```python
from build123d import *

# Parameters (mm, degrees)
SKETCH1_W           = 228.6
SKETCH1_H           = 149.86
SKETCH1_R           = 2.54
SKETCH1_R_2         = 2.159
SKETCH1_W_2         = 25.4
SKETCH1_H_2         = 3.175
BOSS_EXTRUDE1_DEPTH = 2.6
FILLET1_R           = 10
SKETCH6_R           = 2.159
CUT_EXTRUDE6_DEPTH  = 2.6
SKETCH15_R          = 10
CUT_EXTRUDE14_DEPTH = 274.354604132
SKETCH25_W          = 104.14
SKETCH25_H          = 22.86
SKETCH25_W_2        = 3.2385
SKETCH25_H_2        = 12.7
CUT_EXTRUDE18_DEPTH = 10.16


with BuildPart() as part:
    # Sketch1 → Boss-Extrude1 (new body)
    with BuildSketch(Plane(origin=(0, 0, 0), x_dir=(1, 0, 0), z_dir=(0, 1, 0))):
        with Locations((114.3, -74.93)):
            Rectangle(SKETCH1_W, SKETCH1_H)
        with Locations(Location((5.08, -57.785, 0), (0, 0, 270))):
            Circle(SKETCH1_R, mode=Mode.SUBTRACT)
        with Locations(Location((5.08, -92.075, 0), (0, 0, 270))):
            Circle(SKETCH1_R, mode=Mode.SUBTRACT)
        with Locations(Location((223.52, -92.075, 0), (0, 0, 270))):
            Circle(SKETCH1_R, mode=Mode.SUBTRACT)
        with Locations(Location((223.52, -57.785, 0), (0, 0, 270))):
            Circle(SKETCH1_R, mode=Mode.SUBTRACT)
        with Locations(Location((218.44, -10.16, 0), (0, 0, 270))):
            Circle(SKETCH1_R_2, mode=Mode.SUBTRACT)
        with Locations(Location((10.16, -10.16, 0), (0, 0, 270))):
            Circle(SKETCH1_R_2, mode=Mode.SUBTRACT)
        with Locations(Location((218.44, -139.7, 0), (0, 0, 270))):
            Circle(SKETCH1_R_2, mode=Mode.SUBTRACT)
        with Locations(Location((10.16, -139.7, 0), (0, 0, 270))):
            Circle(SKETCH1_R_2, mode=Mode.SUBTRACT)
        with Locations((35.56, -9.887961988)):
            Rectangle(SKETCH1_W_2, SKETCH1_H_2, mode=Mode.SUBTRACT)
        with Locations((193.04, -9.887961988)):
            Rectangle(SKETCH1_W_2, SKETCH1_H_2, mode=Mode.SUBTRACT)
        with Locations((193.04, -139.972038012)):
            Rectangle(SKETCH1_W_2, SKETCH1_H_2, mode=Mode.SUBTRACT)
        with Locations((35.56, -139.972038012)):
            Rectangle(SKETCH1_W_2, SKETCH1_H_2, mode=Mode.SUBTRACT)
    extrude(amount=BOSS_EXTRUDE1_DEPTH)

    # Fillet1
    fillet1_edges = [part.edges().sort_by_distance(p)[0] for p in [
        (0, 1.3, 0),
        (228.6, 1.3, 0),
        (228.6, 1.3, 149.86),
        (0, 1.3, 149.86),
    ]]
    fillet(fillet1_edges, radius=FILLET1_R)

    # Sketch6 → Cut-Extrude6 (cut)
    with BuildSketch(Plane.XZ):
        with Locations((218.6, 10)):
            Circle(SKETCH6_R)
    extrude(amount=-CUT_EXTRUDE6_DEPTH, mode=Mode.SUBTRACT)

    # Sketch15 → Cut-Extrude14 (cut, through all)
    with BuildSketch(Plane.XZ):
        with Locations(Location((114.3, 74.93, 0), (0, 0, 270))):
            Circle(SKETCH15_R)
    extrude(amount=-CUT_EXTRUDE14_DEPTH, mode=Mode.SUBTRACT)

    # Sketch25 → Cut-Extrude18 (cut)
    with BuildSketch(Plane(origin=(0, 2.6, 0), x_dir=(1, 0, 0), z_dir=(0, 1, 0))):
        with Locations((114.3, -74.93)):
            Rectangle(SKETCH25_W, SKETCH25_H)
        with Locations((10.991446919, -53.364023976)):
            Rectangle(SKETCH25_W_2, SKETCH25_H_2)
        with Locations((58.908546919, -54.507023976)):
            Rectangle(SKETCH25_W_2, SKETCH25_H_2)
        with Locations((15.741246919, -105.294323976)):
            Rectangle(SKETCH25_W_2, SKETCH25_H_2)
        with Locations((43.668546919, -105.294323976)):
            Rectangle(SKETCH25_W_2, SKETCH25_H_2)
    extrude(amount=-CUT_EXTRUDE18_DEPTH, mode=Mode.SUBTRACT)


solid = part.part
```
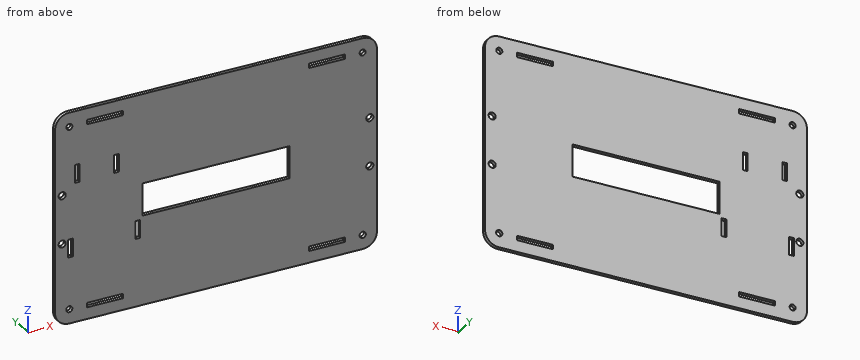
Design review of the part built by this model. Coordinates are the model's own, in mm. Coordinates: 2 decimals unless noted, no trailing zeros. Loops run counter-clockwise (first coordinate to the right, second up) from the corner with the lowest first, then second, coordinate; pieces in that order, holes last. Notation, with made-up numbers: M 71.5,-38 L 86.5,-38 A30 ccw 86.5,-3 Z; hole C 64,4.5 d3. An arc over 180 degrees is marked long. One line per question, with ' | ' between items.
(1) Wall thickness on probe 1 along Z at (x, y) = (188, 1.95); probe 2 along X at (y, z) = (2.25, 103.5); probe 3 along X at (y, z) = (1.1, 139.7): over which ranges is each line inside the solid? List them lowest first.
Filled in:
probe 1: z = 0 to 8.3, 11.48 to 138.38, 141.56 to 149.86 | probe 2: x = 0 to 14.12, 17.36 to 42.05, 45.29 to 228.6 | probe 3: x = 0 to 8, 12.32 to 22.86, 48.26 to 180.34, 205.74 to 216.28, 220.6 to 228.6
(2) We need section B-B (x = 137). Give the boundary of the cut face in (y, z), and give its area (3 significant figures).
Filled in:
outline: M 0,0 L 2.6,0 L 2.6,63.5 L 0,63.5 Z; M 0,86.36 L 2.6,86.36 L 2.6,149.86 L 0,149.86 Z | area: 330 mm^2
(3) For pin 1 Ø8 at (x, z) = (5.08, 57.785) entering from +Y, flat-tipped, find the tip position at first contact; note if it passes through.
Filled in:
pin 1: stops at y = 2.6
(4) We need section D-D (x = 5.08). Give the boundary of the cut face in (y, z) (3 decimals), and give its area (3 significant figures).
Filled in:
outline: M 0,1.294 L 2.6,1.294 L 2.6,55.245 L 0,55.245 Z; M 0,60.325 L 2.6,60.325 L 2.6,89.535 L 0,89.535 Z; M 0,94.615 L 2.6,94.615 L 2.6,148.566 L 0,148.566 Z | area: 356 mm^2
(5) We need section A-A (z = 104.5). Give the boundary of the cut face in (x, y).
Filled in:
outline: M 0,0 L 14.12,0 L 14.12,2.6 L 0,2.6 Z; M 17.36,0 L 42.05,0 L 42.05,2.6 L 17.36,2.6 Z; M 45.29,0 L 228.6,0 L 228.6,2.6 L 45.29,2.6 Z
(6) We need section C-C (z = 81.5). Give the boundary of the cut face in (x, y).
Filled in:
outline: M 0,0 L 62.23,0 L 62.23,2.6 L 0,2.6 Z; M 166.37,0 L 228.6,0 L 228.6,2.6 L 166.37,2.6 Z
